from build123d import *

# Parameters (mm, degrees)
BOX_W           = 62.78
BOX_H           = 108
BOX_DEPTH       = 17.3
SKETCH_W        = 58.78
SKETCH_H        = 104
POCKET_DEPTH    = 15.3
SKETCH001_W     = 2.23
SKETCH001_H     = 31.5
POCKET001_DEPTH = 13
SKETCH002_R     = 3.5
PAD_DEPTH       = 14.5
SKETCH003_R     = 2.5
PAD001_DEPTH    = 0.8


with BuildPart() as part:
    # Box → Box (new body)
    with BuildSketch(Plane.XY):
        with Locations((31.39, 54)):
            Rectangle(BOX_W, BOX_H)
    extrude(amount=BOX_DEPTH)

    # Sketch (on Face6 of Box) → Pocket (cut)
    with BuildSketch(Plane.XY.offset(17.3)):
        with Locations((31.651668, 53.986192)):
            Rectangle(SKETCH_W, SKETCH_H)
    extrude(amount=-POCKET_DEPTH, mode=Mode.SUBTRACT)

    # Sketch001 (on Face3 of Pocket) → Pocket001 (cut)
    with BuildSketch(Plane.XY.offset(17.3)):
        with Locations((61.972029, 74.75)):
            Rectangle(SKETCH001_W, SKETCH001_H)
    extrude(amount=-POCKET001_DEPTH, mode=Mode.SUBTRACT)

    # Sketch002 (on Face14 of Pocket001) → Pad (join)
    with BuildSketch(Plane.XY.offset(2)):
        with Locations((7, 101)):
            Circle(SKETCH002_R)
        with Locations((47, 101)):
            Circle(SKETCH002_R)
        with Locations((7, 7)):
            Circle(SKETCH002_R)
        with Locations((47, 7)):
            Circle(SKETCH002_R)
    extrude(amount=PAD_DEPTH)

    # Sketch003 (on Face20 of Pad) → Pad001 (join)
    with BuildSketch(Plane.XY.offset(16.5)):
        with Locations((7, 7)):
            Circle(SKETCH003_R)
        with Locations((47, 7)):
            Circle(SKETCH003_R)
        with Locations((7, 101)):
            Circle(SKETCH003_R)
        with Locations((47, 101)):
            Circle(SKETCH003_R)
    extrude(amount=PAD001_DEPTH)


solid = part.part
Check sheet for the modelled part. Datum: model origin and axes. Units: mm. A direction names the side the tool comes from. Give positions to 0.01 mm unless a question says otherwise; leave off trailing zeros. Write each loop counter-clockwise with the first axis right and the second up, starting at its lowest first coordinate (ties: lowest second). Pieces come first, ordered by that corner, then holes. Notation, with made-up numbers: (21.25, -29.5) -> (70.25, -29.5) arc R21 cw to (70.25, 6.5) -> close; hole circle Ø1 at (6, -20). An arc over 180 degrees is marked (long way). One line per item, written item: value. Start each with the question number.
Item 1: Section check B-B on x = 7. Record the cut outline in (y, z).
Item 2: Tool access check on faces 5 (the flat face through (47, 7, 17.3)), 6 (the flat face through (49, 5, 16.5)). Record the directions out of +Z, -Z, +X, -X, +Y, -Y that give a thin tool (end or side, any length) a straight path to the whole face; none if there is none.
Item 3: Draft check along X on faces 1 (the flat face through (0, 53, 9)), 2 (the flat face through (62.78, 41, 9)), 3 (the flat face through (31, 55, 2)), 4 (the flat face through (31, 108, 9)). Enter one of: +X half, -X half, draft (parallel to the pull), parting line (faces both ways), or undercut.
Item 4: Material ranges on probe 1 along Y at (x, z) = (20.5, 2.75); probe 2 along X at (y, z) = (48, 5.5); probe 3 along X at (y, z) = (9, 3.5), recorded low to high. Write a range as from..to.
Item 5: Gauge pin test, flat ends, axial feed: pin 1 (0.5 mm diameter, centred on x = 62, y = 71.5, fed in from +Z); pin 2 (8 mm diameter, centred on x = 8, y = 66.5, fed in from +Z). Record the tip position at first contact, or that the pin passes through.
Item 6: Section check C-C on y = 7. Record the cut outline in (x, z), then the cut area to 3 significant figures.
Item 7: Section check A-A on z = 13.5. Record the cut outline in (x, y), then the cut area to 3 significant figures.
Item 8: Section check D-D on y = 87.5. Record the cut outline in (x, z).
Results list:
1. outline: (0, 0) -> (108, 0) -> (108, 17.3) -> (105.99, 17.3) -> (105.99, 2) -> (104.5, 2) -> (104.5, 16.5) -> (103.5, 16.5) -> (103.5, 17.3) -> (98.5, 17.3) -> (98.5, 16.5) -> (97.5, 16.5) -> (97.5, 2) -> (10.5, 2) -> (10.5, 16.5) -> (9.5, 16.5) -> (9.5, 17.3) -> (4.5, 17.3) -> (4.5, 16.5) -> (3.5, 16.5) -> (3.5, 2) -> (1.99, 2) -> (1.99, 17.3) -> (0, 17.3) -> close
2. face 5: +Z, +X, -X, +Y, -Y
2. face 6: +Z
3. face 1: -X half
3. face 2: +X half
3. face 3: undercut
3. face 4: draft
4. probe 1: 0..1.99, 105.99..108
4. probe 2: 0..2.26, 61.04..62.78
4. probe 3: 0..2.26, 4.13..9.87, 44.13..49.87, 61.04..62.78
5. pin 1: z = 4.3
5. pin 2: z = 2
6. outline: (0, 0) -> (62.78, 0) -> (62.78, 17.3) -> (61.04, 17.3) -> (61.04, 2) -> (50.5, 2) -> (50.5, 16.5) -> (49.5, 16.5) -> (49.5, 17.3) -> (44.5, 17.3) -> (44.5, 16.5) -> (43.5, 16.5) -> (43.5, 2) -> (10.5, 2) -> (10.5, 16.5) -> (9.5, 16.5) -> (9.5, 17.3) -> (4.5, 17.3) -> (4.5, 16.5) -> (3.5, 16.5) -> (3.5, 2) -> (2.26, 2) -> (2.26, 17.3) -> (0, 17.3) -> close
6. area: 398 mm²
7. outline: (0, 0) -> (62.78, 0) -> (62.78, 59) -> (61.04, 59) -> (61.04, 1.99) -> (2.26, 1.99) -> (2.26, 105.99) -> (61.04, 105.99) -> (61.04, 90.5) -> (62.78, 90.5) -> (62.78, 108) -> (0, 108) -> close; circle Ø7 at (7, 7); circle Ø7 at (7, 101); circle Ø7 at (47, 7); circle Ø7 at (47, 101)
7. area: 766 mm²
8. outline: (0, 0) -> (62.78, 0) -> (62.78, 4.3) -> (61.04, 4.3) -> (61.04, 2) -> (2.26, 2) -> (2.26, 17.3) -> (0, 17.3) -> close
